Verification items for the finished model (mm, model axes). A direction names the side the tool comes from. Coordinates: 2 decimals unless noted, no trailing zeros. Write each loop counter-clockwise with the first axis right and the second up, starting at its lowest first coordinate (ties: lowest second). Pieces come first, ordered by that corner, then holes. Notation, with made-up numbers: (14.5, -40) -> (21.5, -40) arc R18 cw to (21.5, -19) -> close; hole circle Ø8 at (29.25, 30.25). An arc over 180 degrees is marked (long way). Write item = value, one per line. Start each with the question number.
(1) Material ranges on probe 1 along Z at (x, y) = (-25.5, -82); probe 2 along Y at (x, z) = (84.5, 158); probe 3 along Z at (x, y) = (-9.5, 47), recorded low to high. Write a range as [from, to].
(2) Section check C-C (x = -10.5). Record the cut outline in (y, z), plus the area to 3 significant figures.
(3) Section check D-D (z = 88.9). Record the cut outline in (x, y).
(4) Set-up check for faces 1 (the face through (37, 18, 0)), 2 (the face through (0.082, -58, 139)), 3 (the face through (29.372, -156.776, 49.226)): record each of +Z, -Z, +X, -X, +Y, -Y from which the full face is reachable in a straight line by a thin tool's end or side.
(5) Section check A-A (z = 36.5). Record the cut outline in (x, y), plus the area to 3 significant figures.
(6) Section check B-B (y = 22). Record the cut outline in (x, z).
(7) Gauge pin test, flat ends, axial feed: pin 1 Ø10 at (y, z) = (-171, 135) entering from +X; pin 2 Ø3 at (x, z) = (70.5, 106.5) entering from -Y; pin 3 Ø1 at (x, y) = (51, -23) entering from +Z; pin 4 Ø8 at (x, z) = (94, 34) entering from -Y. Record the tip position at first contact, or that the pin passes through.
(8) Mould release check, pull along Y, two halves, no side actions. Record for faces 4 (the face through (19.461, 71.645, 37.922)), 5 (the face through (37.649, -60.543, 126.289)), 6 (the face through (49.1, 43.5, 50.8)): released by +Y, released by -Y, zero draft, split by the parting line, or undercut.
```python
from build123d import *

# Parameters (mm, degrees)
F0_R      = 25.4
F0_R_2    = 15.24
F1_DEPTH  = 50.8
F2_DEPTH  = 25.4
F0_W      = 152.4
F0_H      = 50.8
F3_DEPTH  = 177.8
F4_R      = 40.64
F5_DEPTH  = 127
F6_R      = 7.62
F9_DEPTH  = 164.846
F10_DEPTH = 38.1
F11_DEPTH = 38.1
F12_R     = 12.7


with BuildPart() as f1:
    # F0 (on Top) → F1 (new body)
    with BuildSketch(Plane.XY):
        with Locations((38.1820415974, 54.4787267387)):
            Circle(F0_R)
        with Locations((38.1820415974, 54.4787267387)):
            Circle(F0_R_2, mode=Mode.SUBTRACT)
    extrude(amount=F1_DEPTH)

    # F0 (on Top) → F2 (join)
    with BuildSketch(Plane.XY):
        with BuildLine():
            Line((114.3820415974, -47.1212732613), (114.3820415974, 54.4787267387))
            ThreePointArc((114.3820415974, 54.4787267387), (92.0635783238, 108.3602634651), (38.1820415974, 130.6787267387))
            ThreePointArc((38.1820415974, 130.6787267387), (-15.699495129, 108.3602634651), (-38.0179584026, 54.4787267387))
            Line((-38.0179584026, 54.4787267387), (-38.0179584026, -47.1212732613))
            Line((-38.0179584026, -47.1212732613), (114.3820415974, -47.1212732613))
        make_face()
        with Locations((38.1820415974, 54.4787267387)):
            Circle(F0_R, mode=Mode.SUBTRACT)
    extrude(amount=F2_DEPTH)

    # F0 (on Top) → F3 (join)
    with BuildSketch(Plane.XY):
        with Locations((38.1820415974, -72.5212732613)):
            Rectangle(F0_W, F0_H)
    extrude(amount=F3_DEPTH)

    # F4 (on face) → F5 (join)
    with BuildSketch(Plane.XZ.offset(97.9212732613)):
        with Locations((38.1820415974, 88.9)):
            Circle(F4_R)
    extrude(amount=F5_DEPTH)

    # F6
    f6_edges = [f1.edges().sort_by_distance(p)[0] for p in [
        (-2.457958, -224.921273, 88.9),
    ]]
    fillet(f6_edges, radius=F6_R)

    # F8 (on face) → F9 (cut)
    with BuildSketch(Plane(origin=(-38.0179584026, 0, 0), x_dir=(0, -1, 0), z_dir=(-1, 0, 0))):
        Polygon((74.3449112123, 177.8), (47.1212732613, 177.8), (47.1212732613, 76.2), align=None)
    extrude(amount=-F9_DEPTH, mode=Mode.SUBTRACT)

    # F7 (on face) → F10 (join)
    with BuildSketch(Plane.YZ.offset(114.3820415974)):
        Polygon((-47.1212732613, 25.4), (-47.1212732613, 76.2), (-74.3449112123, 177.8), (-97.9212732613, 177.8), (-97.9212732613, 0), (54.4787267387, 0), (54.4787267387, 25.4), align=None)
        Polygon((-47.1212732613, 76.2), (-47.1212732613, 177.8), (-74.3449112123, 177.8), align=None)
    extrude(amount=-F10_DEPTH)

    # F8 (on face) → F11 (join)
    with BuildSketch(Plane(origin=(-38.0179584026, 0, 0), x_dir=(0, -1, 0), z_dir=(-1, 0, 0))):
        Polygon((74.3449112123, 177.8), (47.1212732613, 177.8), (47.1212732613, 76.2), align=None)
        Polygon((74.3449112123, 177.8), (47.1212732613, 76.2), (47.1212732613, 25.4), (-54.4787267387, 25.4), (-54.4787267387, 0), (97.9212732613, 0), (97.9212732613, 177.8), align=None)
    extrude(amount=-F11_DEPTH)

    # F12
    f12_edges = [f1.edges().sort_by_distance(p)[0] for p in [
        (114.382042, -72.521273, 177.8),
        (-38.017958, -72.521273, 177.8),
    ]]
    fillet(f12_edges, radius=F12_R)


solid = f1.part
```
Response:
q1.probe_1 = [0, 177.8]
q1.probe_2 = [-97.92, -47.12]
q1.probe_3 = [0, 25.4]
q2.outline = (-97.92, 0) -> (113.1, 0) -> (113.1, 25.4) -> (-47.12, 25.4) -> (-47.12, 177.8) -> (-97.92, 177.8) -> close
q2.area = 13,100 mm2
q3.outline = (-38.02, -97.92) -> (-2.46, -97.92) -> (-2.46, -217.3) arc R7.62 ccw to (5.16, -224.92) -> (71.2, -224.92) arc R7.62 ccw to (78.82, -217.3) -> (78.82, -97.92) -> (114.38, -97.92) -> (114.38, -47.12) -> (76.28, -47.12) -> (76.28, -50.52) -> (0.08, -50.52) -> (0.08, -47.12) -> (-38.02, -47.12) -> close
q4.face_1 = -Z, +X, -X, +Y, -Y
q4.face_2 = +Z, +Y
q4.face_3 = -Y
q5.outline = (-38.02, -97.92) -> (114.38, -97.92) -> (114.38, -47.12) -> (-38.02, -47.12) -> close; circle Ø50.8 at (38.18, 54.48); hole circle Ø30.48 at (38.18, 54.48)
q5.area = 9,040 mm2
q6.outline = (-38.02, 0) -> (114.38, 0) -> (114.38, 25.4) -> (-38.02, 25.4) -> close
q7.pin_1 = through
q7.pin_2 = -224.57
q7.pin_3 = 25.4
q7.pin_4 = -97.92
q8.face_4 = undercut
q8.face_5 = released by +Y
q8.face_6 = zero draft
